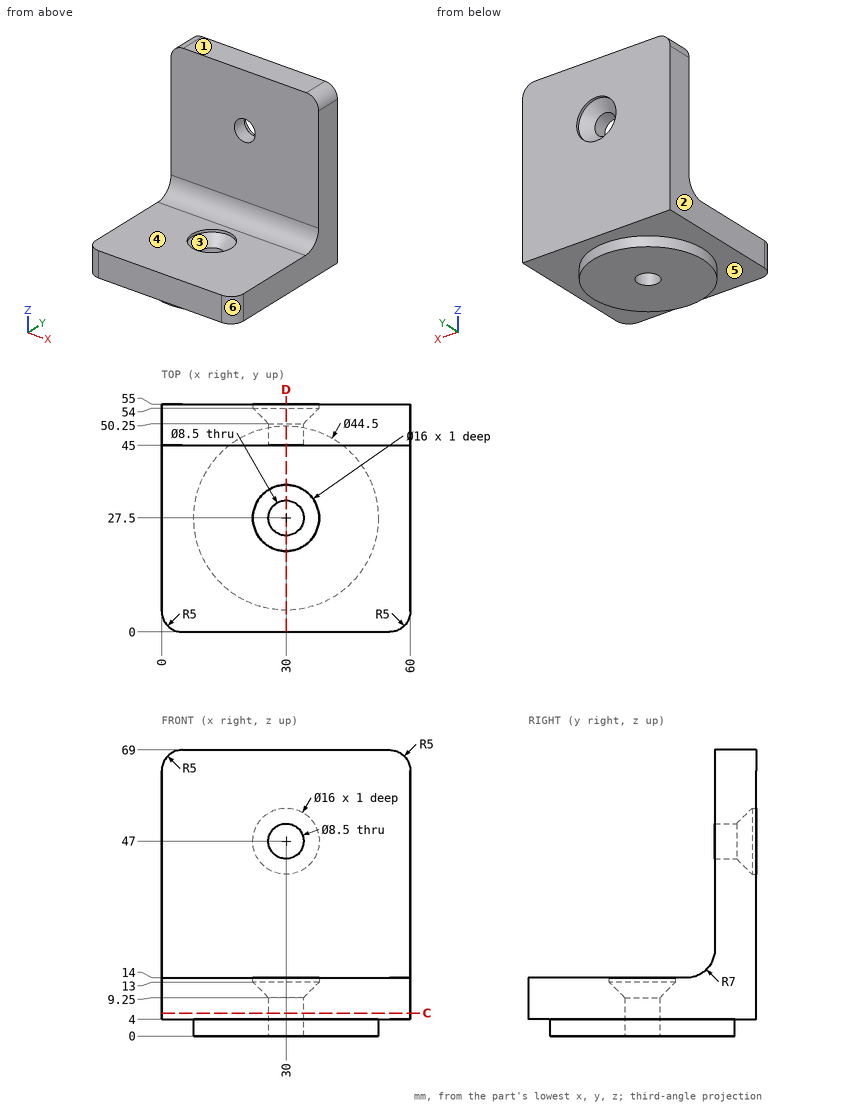
Input: dimensioned drawing with shaded views. Units: mm. Origin: part minimum x, y, z. A direction names the side the tool comes from. Give positions to 0.01 mm unless a question says otherwise; leave off trailing zeros. Write each loop counter-clockwise with the first axis right and the second up, starting at its lowest first coordinate (ties: lowest second). Pieces come first, ordered by that corner, then holes. Notation, with made-up numbers: (51.25, 20) -> (79.25, 20) arc R20 ccw to (79.25, 25) -> close; hole circle Ø6 at (-8, 68). An arc over 180 degrees is marked (long way). Return JSON: item names as keys, results as strings. Group by question number.
1. Section C-C, the plane z = 5.5. Output: boundary loops of the cut face in (x, y).
2. Mould query, pull axis X, two halves, no side actions, for the marked faces 1, 2 and 3. Classes: +X half, -X half, draft (parallel to the pull), parting line (faces both ways), or undercut.
3. Pin query (flat end, axial travel): pin 1 Ø3 at (x, z) = (8, 30.5) entering from -Y; pin 2 Ø8 at (x, y) = (13.5, 23) entering from +Z; pin 3 Ø6 at (x, y) = (8.5, 47.5) entering from -Z. Return the tip coordinate at first contact, or that it passes through.
4. Section D-D, the plane x = 30. Count the separate pieces of the cut face and the enclosed holes in it, then the cut area to 3 significant figures.
5. Material intervals for line 1 (Z direction, x = 30, y = 46); line 2 (X direction, y = 27.5, z = 5.5); line 3 (Z direction, x = 30, y = 54), sorted ascending. Write a range as from..to.
6. Access query for the marked faces 4, 5 and 6. Directions: +Z, -Z, +X, -X, +Y, -Y. A direction counts if a zero-diameter tool reaches every point of the face in a straight line with its end or side. Return the directions, or none.
Determined:
{
 "1": {"outline": "(0, 5) arc R5 ccw to (5, 0) -> (55, 0) arc R5 ccw to (60, 5) -> (60, 55) -> (0, 55) -> close; hole circle Ø8.5 at (30, 27.5)"},
 "2": {"face 1": "draft", "face 2": "-X half", "face 3": "undercut"},
 "3": {"pin 1": "stops at y = 45", "pin 2": "stops at z = 14", "pin 3": "stops at z = 4"},
 "4": {"separate pieces": "3", "enclosed holes": "0", "area": "1,040 mm2"},
 "5": {"line 1": "z = 0..42.75, 51.25..69", "line 2": "x = 0..25.75, 34.25..60", "line 3": "z = 4..39, 55..69"},
 "6": {"face 4": "+Z, +X, -X, -Y", "face 5": "-Z", "face 6": "+Z, -Z, +X, -Y"}
}
